Geometry: see drawing. Coordinates: mm, zero at the bounding-box minimum. A direction names the side the tool comes from. Round coordinates to 2 decimals unless told otherwise and drop trailing zeros. Loops run counter-clockwise (first coordinate to the right, second up) from the corner with the lowest first, then second, coordinate; pieces in that order, holes last. Notation, with made-up numbers: (54.5, -38) -> (83.5, -38) arc R19 ccw to (83.5, -2) -> close; hole circle Ø1 at (-9.5, 13). An arc over 180 degrees is marked (long way). Write item = value, one per line.
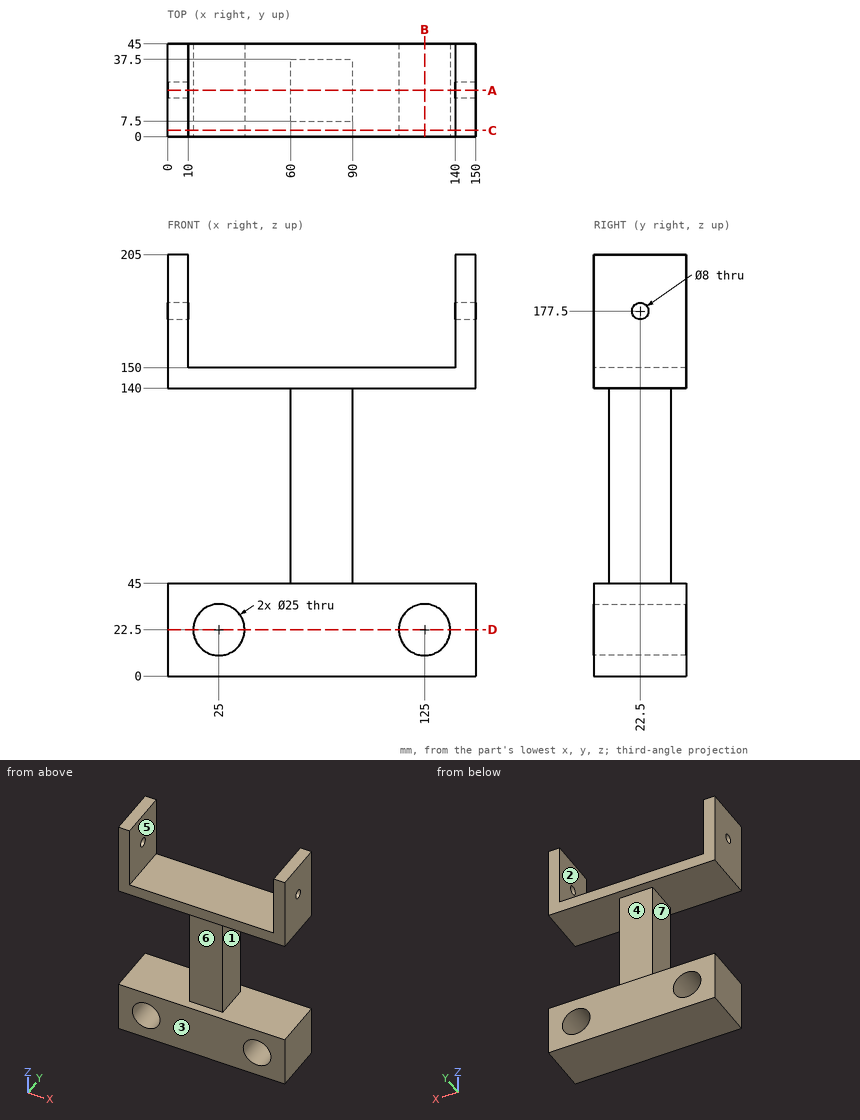
1. Contact query for flat-ended pins moving along their axis: pin 1 Ø15 at (x, z) = (70, 90.5) entering from -Y; pin 2 Ø3 at (x, y) = (126, 19) entering from -Z; pin 3 Ø15 at (x, z) = (25, 22.5) entering from -Y; pin 4 Ø9 at (y, z) = (16.5, 93.5) entering from +X. Output: stop coordinate, or through.
Evaluation:
pin_1 = 7.5
pin_2 = 0
pin_3 = through
pin_4 = 90
2. Section query D-D (z = 22.5). Return the cut outline in (x, y), then the cut area to 3 significant figures.
Evaluation:
outline = (0, 0) -> (12.5, 0) -> (12.5, 45) -> (0, 45) -> close; (37.5, 0) -> (112.5, 0) -> (112.5, 45) -> (37.5, 45) -> close; (137.5, 0) -> (150, 0) -> (150, 45) -> (137.5, 45) -> close
area = 4,500 mm²
3. Section query B-B (x = 125). Return the cut outline in (y, z).
Evaluation:
outline = (0, 0) -> (45, 0) -> (45, 10) -> (0, 10) -> close; (0, 35) -> (45, 35) -> (45, 45) -> (0, 45) -> close; (0, 140) -> (45, 140) -> (45, 150) -> (0, 150) -> close
4. Line query: probe 1 along Z at (x, y) = (125, 20); probe 2 along Z at (x, y) = (4, 22.5); probe 3 along X at (y, z) = (33, 22). Output: solid intervals per line, ascending. Write a range as from..to.
Evaluation:
probe_1 = 0..10, 35..45, 140..150
probe_2 = 0..45, 140..173.5, 181.5..205
probe_3 = 0..12.51, 37.49..112.51, 137.49..150
5. Section query C-C (y = 3). Return the cut outline in (x, z), then the cut area to 3 significant figures.
Evaluation:
outline = (0, 0) -> (150, 0) -> (150, 45) -> (0, 45) -> close; (0, 140) -> (150, 140) -> (150, 205) -> (140, 205) -> (140, 150) -> (10, 150) -> (10, 205) -> (0, 205) -> close; hole circle Ø25 at (25, 22.5); hole circle Ø25 at (125, 22.5)
area = 8,370 mm²
6. Section query A-A (y = 22.5). Return the cut outline in (x, z).
Evaluation:
outline = (0, 0) -> (150, 0) -> (150, 45) -> (90, 45) -> (90, 140) -> (150, 140) -> (150, 173.5) -> (140, 173.5) -> (140, 150) -> (10, 150) -> (10, 173.5) -> (0, 173.5) -> (0, 140) -> (60, 140) -> (60, 45) -> (0, 45) -> close; (0, 181.5) -> (10, 181.5) -> (10, 205) -> (0, 205) -> close; (140, 181.5) -> (150, 181.5) -> (150, 205) -> (140, 205) -> close; hole circle Ø25 at (25, 22.5); hole circle Ø25 at (125, 22.5)
7. Set-up query: the marked faces 4, 5, 6 and 7. Return all of +Z, -Z, +X, -X, +Y, -Y with unobstructed straight access to the full face (end or side cutting, diameter ignored); none if empty.
Evaluation:
face_4 = +X, -X, +Y
face_5 = +Z, +Y, -Y
face_6 = +X, -X, -Y
face_7 = -X, +Y, -Y
8. Mould query, pull axis X, two halves, no side actions, for the marked faces 1, 2 and 3. Classes: released by +X, released by -X, zero draft, split by the parting line, or undercut.
Evaluation:
face_1 = released by +X
face_2 = undercut
face_3 = zero draft
